Read the model definition and answer for the solid it produces. Units are mm, in the model's axes. A direction names the side the tool comes from. Coordinates: 2 decimals unless noted, no trailing zeros. Loops run counter-clockwise (first coordinate to the right, second up) from the corner with the lowest first, then second, coordinate; pieces in that order, holes last.
from build123d import *

# Parameters (mm, degrees)
SKETCH_1_R      = 1.15
EXTRUDE_1_DEPTH = 2
FILLET_1_R      = 6
FILLET_2_R      = 6
FILLET_3_R      = 2


with BuildPart() as part:
    # Эскиз1 → Бобышка-Вытянуть1 (new body)
    with BuildSketch(Plane(origin=(0, 0, 0), x_dir=(1, 0, 0), z_dir=(0, 1, 0))):
        with BuildLine():
            Line((2.236067977, -2), (16.605931339, -2))
            ThreePointArc((16.605931339, -2), (19.434358463, 0), (22.262785588, -2))
            Line((22.262785588, -2), (28.713932023, -2))
            ThreePointArc((28.713932023, -2), (33.95, 0), (28.713932023, 2))
            Line((28.713932023, 2), (24.333337949, 2))
            ThreePointArc((24.333337949, 2), (19.434358463, 4), (14.535378978, 2))
            Line((14.535378978, 2), (2.236067977, 2))
            ThreePointArc((2.236067977, 2), (-3, 0), (2.236067977, -2))
        make_face()
        with Locations(Location((0, 0, 0), (0, 0, 270))):
            Circle(SKETCH_1_R, mode=Mode.SUBTRACT)
        with Locations(Location((30.95, 0, 0), (0, 0, 270))):
            Circle(SKETCH_1_R, mode=Mode.SUBTRACT)
    extrude(amount=EXTRUDE_1_DEPTH)

    # Скругление1
    fillet_1_edges = [part.edges().sort_by_distance(p)[0] for p in [
        (2.236067977, 1, 2),
        (2.236067977, 1, -2),
        (28.713932023, 1, -2),
        (28.713932023, 1, 2),
    ]]
    fillet(fillet_1_edges, radius=FILLET_1_R)

    # Скругление2
    fillet_2_edges = [part.edges().sort_by_distance(p)[0] for p in [
        (22.262785588, 1, 2),
        (16.605931339, 1, 2),
    ]]
    fillet(fillet_2_edges, radius=FILLET_2_R)

    # Скругление3
    fillet_3_edges = [part.edges().sort_by_distance(p)[0] for p in [
        (14.535378978, 1, -2),
        (24.333337949, 1, -2),
    ]]
    fillet(fillet_3_edges, radius=FILLET_3_R)


solid = part.part
Item 1: A cutting plane is placed at A-A on x = 0. Determine the outline of the cut face in (y, z).
Numbers:
outline: (0, -3) - (2, -3) - (2, -1.15) - (0, -1.15) - close; (0, 1.15) - (2, 1.15) - (2, 3) - (0, 3) - close
Item 2: Which of the six approach directions +Z, -Z, +X, -X, +Y, -Y give full straight-line access (tool end or side, diameter ignored) to faces 3 (the face through (28.261, 1.014, -2.174)), 4 (the face through (15.751, 1.014, 1.666)), 5 (the face through (-3, 1, 0))?
Numbers:
face 3: -Z, +Y, -Y
face 4: +Z, +Y, -Y
face 5: +Y, -Y
Item 3: Determine the mould class of faces 1 (the face through (15, 2, -1)), 2 (the face through (14.4, 1, -2.1)) for opening direction X: released by +X, released by -X, zero draft, split by the parting line, or undercut.
Numbers:
face 1: zero draft
face 2: undercut
Item 4: Given pin 1 (0.9 mm diameter, centred on x = 26, y = 1, fed in from -Z); pin 2 (0.9 mm diameter, centred on x = 26, y = 1.5, fed in from +Z); pin 3 (1.8 mm diameter, centred on x = 0, z = 0, fed in from +Y); pin 4 (1 mm diameter, centred on y = 1.5, z = -3, fed in from -X), each flat-ended and moving along its own axis, determine where each tip first touches the part or whether it passes through.
Numbers:
pin 1: stops at z = -2
pin 2: stops at z = 2
pin 3: passes through
pin 4: stops at x = -1.66
Item 5: A cutting plane is placed at B-B on y = 1.65. Determine the outline of the cut face in (x, z).
Numbers:
outline: (1.37, -2.67) arc R6 cw to (4.12, -2) - (13.78, -2) arc R2 cw to (15.03, -2.44) arc R7 ccw to (23.83, -2.44) arc R2 cw to (25.09, -2) - (26.83, -2) arc R6 cw to (29.58, -2.67) arc R3 ccw (long way) to (29.58, 2.67) arc R6 cw to (26.83, 2) - (25.09, 2) arc R6 ccw to (21.32, 0.67) arc R3 cw to (17.55, 0.67) arc R6 ccw to (13.78, 2) - (4.12, 2) arc R6 cw to (1.37, 2.67) arc R3 ccw (long way) to start; hole circle Ø2.3 at (0, 0); hole circle Ø2.3 at (30.95, 0)
Item 6: A cutting plane is placed at C-C on z = 1.5. Determine the outline of the cut face in (x, y), then the cut area to 3 significant figures.
Numbers:
outline: (-2.6, 0) - (16.18, 0) - (16.18, 2) - (-2.6, 2) - close; (22.69, 0) - (33.55, 0) - (33.55, 2) - (22.69, 2) - close
area: 59.3 mm2
Item 7: A cutting plane is placed at D-D on x = 10. Determine the outline of the cut face in (y, z), then the cut area to 3 significant figures.
Numbers:
outline: (0, -2) - (2, -2) - (2, 2) - (0, 2) - close
area: 8.00 mm2
Item 8: Find the intervals of material crossed by line 1 along X through (y, z) = (1.75, 0.5); line 2 along Z through (x, y) = (6, 1.15); line 3 along X through (y, z) = (0.1, -0.25), in increasing order.
Numbers:
line 1: x = -2.96 to -1.04, 1.04 to 17.78, 21.09 to 29.91, 31.99 to 33.91
line 2: z = -2 to 2
line 3: x = -2.99 to -1.12, 1.12 to 29.83, 32.07 to 33.94
